The listing builds one solid part. Answer for the finished solid, in the listing's coordinates (mm). A direction names the side the tool comes from. Coordinates: 2 decimals unless noted, no trailing zeros. Loops run counter-clockwise (first coordinate to the right, second up) from the corner with the lowest first, then second, coordinate; pieces in that order, holes last. Notation, with made-up numbers: (79, 34.5) - (119, 34.5) arc R25 cw to (119, 64.5) - close; hole circle Ø9 at (83, 36). An arc over 180 degrees is marked (long way). Put each result on its own line as item: value.
```python
from build123d import *

# Parameters (mm, degrees)
F0_R     = 88.9
F1_DEPTH = 152.4
F4_DEPTH = 152.401
F5_DEPTH = 152.401
F7_DEPTH = 152.401


with BuildPart() as f1:
    # F0 (on Front) → F1 (new body)
    with BuildSketch(Plane.XZ):
        Circle(F0_R)
    extrude(amount=-F1_DEPTH)

    # F3 (on face) → F4 (cut, through all)
    with BuildSketch(Plane.XZ):
        with BuildLine():
            ThreePointArc((6.3453015162, 82.3057692308), (0, 76.2), (-6.3453015162, 82.3057692308))
            ThreePointArc((-6.3453015162, 82.3057692308), (-58.3716647869, 58.3716647869), (-82.3057692308, 6.3453015162))
            ThreePointArc((-82.3057692308, 6.3453015162), (-77.974338005, 4.4029328075), (-76.2, 0))
            ThreePointArc((-76.2, 0), (-77.974338005, -4.4029328075), (-82.3057692308, -6.3453015162))
            ThreePointArc((-82.3057692308, -6.3453015162), (-58.3716647869, -58.3716647869), (-6.3453015162, -82.3057692308))
            ThreePointArc((-6.3453015162, -82.3057692308), (0, -76.2), (6.3453015162, -82.3057692308))
            ThreePointArc((6.3453015162, -82.3057692308), (58.3716647869, -58.3716647869), (82.3057692308, -6.3453015162))
            ThreePointArc((82.3057692308, -6.3453015162), (76.2, 0), (82.3057692308, 6.3453015162))
            ThreePointArc((82.3057692308, 6.3453015162), (58.3716647869, 58.3716647869), (6.3453015162, 82.3057692308))
        make_face()
    extrude(amount=-F4_DEPTH, mode=Mode.SUBTRACT)

    # F2 (on face) → F5 (cut, through all)
    with BuildSketch(Plane.XZ):
        with BuildLine():
            ThreePointArc((-2.7935998838, 82.5027169231), (-1.9588679235, 80.5576966952), (0, 79.756))
            ThreePointArc((0, 79.756), (1.9588679235, 80.5576966952), (2.7935998838, 82.5027169231))
            ThreePointArc((2.7935998838, 82.5027169231), (2.7938999692, 82.5263576151), (2.794, 82.55))
            ThreePointArc((2.794, 82.55), (-0.0236423849, 85.3438999692), (-2.7935998838, 82.5027169231))
        make_face()
        with BuildLine():
            ThreePointArc((-82.5027169231, 2.7935998838), (-85.344, 0), (-82.5027169231, -2.7935998838))
            ThreePointArc((-82.5027169231, -2.7935998838), (-80.5576966952, -1.9588679235), (-79.756, 0))
            ThreePointArc((-79.756, 0), (-80.5576966952, 1.9588679235), (-82.5027169231, 2.7935998838))
        make_face()
        with BuildLine():
            ThreePointArc((79.756, 0), (80.5576966952, -1.9588679235), (82.5027169231, -2.7935998838))
            ThreePointArc((82.5027169231, -2.7935998838), (84.5088679235, -1.9923033048), (85.344, 0))
            ThreePointArc((85.344, 0), (84.5088679235, 1.9923033048), (82.5027169231, 2.7935998838))
            ThreePointArc((82.5027169231, 2.7935998838), (80.5576966952, 1.9588679235), (79.756, 0))
        make_face()
        with BuildLine():
            ThreePointArc((2.794, -82.55), (2.7938999692, -82.5263576151), (2.7935998838, -82.5027169231))
            ThreePointArc((2.7935998838, -82.5027169231), (1.9588679235, -80.5576966952), (0, -79.756))
            ThreePointArc((0, -79.756), (-1.9588679235, -80.5576966952), (-2.7935998838, -82.5027169231))
            ThreePointArc((-2.7935998838, -82.5027169231), (-0.0236423849, -85.3438999692), (2.794, -82.55))
        make_face()
    extrude(amount=-F5_DEPTH, mode=Mode.SUBTRACT)

    # F6 (on face) → F7 (cut, through all)
    with BuildSketch(Plane.XZ):
        with BuildLine():
            Line((82.55, 0), (76.2, 0))
            ThreePointArc((76.2, 0), (77.974338005, -4.4029328075), (82.3057692308, -6.3453015162))
            ThreePointArc((82.3057692308, -6.3453015162), (58.3716647869, -58.3716647869), (6.3453015162, -82.3057692308))
            ThreePointArc((6.3453015162, -82.3057692308), (0, -76.2), (-6.3453015162, -82.3057692308))
            ThreePointArc((-6.3453015162, -82.3057692308), (-58.3716647869, -58.3716647869), (-82.3057692308, -6.3453015162))
            ThreePointArc((-82.3057692308, -6.3453015162), (-77.974338005, -4.4029328075), (-76.2, 0))
            Line((-76.2, 0), (-88.9, 0))
            Line((-88.9, 0), (-104.8936669013, -139.8783236514))
            Line((-104.8936669013, -139.8783236514), (114.9751045783, -122.2419444763))
            Line((114.9751045783, -122.2419444763), (88.9, 0))
            Line((88.9, 0), (82.55, 0))
        make_face()
        Polygon((88.9, 6.35), (88.9, 0), (114.9751045783, -122.2419444763), (179.3332546949, -117.0795708895), (106.4055040479, 6.35), align=None)
        with BuildLine():
            ThreePointArc((82.3057692308, 6.3453015162), (77.974338005, 4.4029328075), (76.2, 0))
            Line((76.2, 0), (82.55, 0))
            Line((82.55, 0), (88.9, 0))
            Line((88.9, 0), (88.9, 6.35))
            Line((88.9, 6.35), (88.138, 6.35))
            ThreePointArc((88.138, 6.35), (85.598, 3.81), (83.058, 6.35))
            Line((83.058, 6.35), (82.55, 6.35))
            Line((82.55, 6.35), (82.3054068698, 6.35))
            ThreePointArc((82.3054068698, 6.35), (82.3055880838, 6.3476507607), (82.3057692308, 6.3453015162))
        make_face()
        with BuildLine():
            Line((-88.9, 0), (-76.2, 0))
            ThreePointArc((-76.2, 0), (-77.974338005, 4.4029328075), (-82.3057692308, 6.3453015162))
            ThreePointArc((-82.3057692308, 6.3453015162), (-82.3055880838, 6.3476507607), (-82.3054068698, 6.35))
            Line((-82.3054068698, 6.35), (-82.55, 6.35))
            Line((-82.55, 6.35), (-83.058, 6.35))
            ThreePointArc((-83.058, 6.35), (-85.598, 3.81), (-88.138, 6.35))
            Line((-88.138, 6.35), (-88.9, 6.35))
            Line((-88.9, 6.35), (-88.9, 0))
        make_face()
    extrude(amount=-F7_DEPTH, mode=Mode.SUBTRACT)

    # F8: F1 across face


with BuildPart() as f1_1:
    add(f1.part)
    add(f1.part.mirror(Plane.XZ))


solid = f1_1.part
```
1) Straight lines are drawn through the part: L1, parallel to X at y = 140, z = 69; L2, parallel to X at y = 124.5, z = 55.5; L3, parallel to Z at x = -29.5, y = 29.5. For each, find the intervals that lie inside material, in ascending order. Write a range as [from, to].
Found:
L1: x = [-56.06, -45.32], [45.32, 56.06]
L2: x = [-69.45, -61.11], [61.11, 69.45]
L3: z = [77.1, 83.86]
2) The part is cut by section B-B (z = 20). Give the vertices of the cut face in (x, y), and give its area (3 significant figures).
Found:
outline: (-86.62, -152.4) - (-80.09, -152.4) - (-80.09, 152.4) - (-86.62, 152.4) - close; (80.09, -152.4) - (86.62, -152.4) - (86.62, 152.4) - (80.09, 152.4) - close
area: 3,980 mm^2
3) The part is cut by section C-C (x = 18.5). Give the vertices of the cut face in (y, z).
Found:
outline: (-152.4, 80.45) - (152.4, 80.45) - (152.4, 86.95) - (-152.4, 86.95) - close
4) For faces 1 (the face through (58.95, 2.13, 57.79)), 2 (the face through (0, -152.4, 78)), determine the directions among +Z, -Z, +X, -X, +Y, -Y from which every point of the face is accessible in a straight line to the end or side of a thin tool.
Found:
face 1: -Z, +Y, -Y
face 2: +Z, -Z, +X, -X, -Y
5) Each of these flat-tipped pins is pushed along its axis until it touches: pin 1 (12 mm diameter, centred on x = -25.5, y = 74, fed in from -Z); pin 2 (6 mm diameter, centred on x = 29.5, y = -87.5, fed in from +Z); pin 3 (2 mm diameter, centred on y = -53.5, z = 26, fed in from +X). Where does it stop, or does it pass through?
Found:
pin 1: stops at z = 76.3
pin 2: stops at z = 84.86
pin 3: stops at x = 85.31
6) The part is cut by section D-D (z = 44). Give the vertices of the cut face in (x, y), and give its area (3 significant figures).
Found:
outline: (-77.25, -152.4) - (-69.85, -152.4) - (-69.85, 152.4) - (-77.25, 152.4) - close; (69.85, -152.4) - (77.25, -152.4) - (77.25, 152.4) - (69.85, 152.4) - close
area: 4,510 mm^2
7) For a pull along X with two mould halves and no side action, classify faces 3 (the face through (-57.79, 2.13, 58.95)), 4 (the face through (1.87, 2.13, 88.88)), 5 (the face through (0, 152.4, 78)), 6 (the face through (0.1, 2.1, 76.2)) as pulls with the +X half, pulls with the -X half, needs draft (parallel to the pull), parting line crosses it, or undercut.
Found:
face 3: undercut
face 4: parting line crosses it
face 5: needs draft
face 6: undercut
8) The part is cut by section A-A (y = -35). Give the vertices of the cut face in (x, z).
Found:
outline: (-88.67, 6.35) - (-88.14, 6.35) arc R2.54 ccw to (-83.06, 6.35) - (-82.31, 6.35) arc R82.55 cw to (-6.35, 82.31) arc R6.35 ccw to (6.35, 82.31) arc R82.55 cw to (82.31, 6.35) - (83.06, 6.35) arc R2.54 ccw to (88.14, 6.35) - (88.67, 6.35) arc R88.9 ccw to start; hole circle Ø5.59 at (0, 82.55)
